from build123d import *

# Parameters (mm, degrees)
SKETCH2_W           = 26
SKETCH2_H           = 11
SKETCH2_W_2         = 20.4
SKETCH2_H_2         = 6.5
BOSS_EXTRUDE1_DEPTH = 10
SKETCH3_W           = 26
SKETCH3_H           = 11
SKETCH3_W_2         = 2.5
SKETCH3_H_2         = 6.5
BOSS_EXTRUDE2_DEPTH = 6
SKETCH4_W           = 11
SKETCH4_H           = 40
SKETCH4_R           = 2.85
BOSS_EXTRUDE3_DEPTH = 6
FILLET1_R           = 2


with BuildPart() as part:
    # Sketch2 → Boss-Extrude1 (new body)
    with BuildSketch(Plane(origin=(0, 0, 0), x_dir=(1, 0, 0), z_dir=(0, 1, 0))):
        Rectangle(SKETCH2_W, SKETCH2_H)
        Rectangle(SKETCH2_W_2, SKETCH2_H_2, mode=Mode.SUBTRACT)
    extrude(amount=BOSS_EXTRUDE1_DEPTH)

    # Sketch3 → Boss-Extrude2 (add)
    with BuildSketch(Plane.XZ):
        Rectangle(SKETCH3_W, SKETCH3_H)
        with Locations((-7.45, 0)):
            Rectangle(SKETCH3_W_2, SKETCH3_H_2, mode=Mode.SUBTRACT)
        with Locations((-0.25, 0)):
            Rectangle(SKETCH3_W_2, SKETCH3_H_2, mode=Mode.SUBTRACT)
        with Locations((7.45, 0)):
            Rectangle(SKETCH3_W_2, SKETCH3_H_2, mode=Mode.SUBTRACT)
    extrude(amount=BOSS_EXTRUDE2_DEPTH)

    # Sketch4 → Boss-Extrude3 (add)
    with BuildSketch(Plane(origin=(13, 0, 0), x_dir=(0, 0, -1), z_dir=(1, 0, 0))):
        with Locations((0, 2)):
            Rectangle(SKETCH4_W, SKETCH4_H)
        with Locations((0, 16)):
            Circle(SKETCH4_R, mode=Mode.SUBTRACT)
        with Locations((0, -11.995757917)):
            Circle(SKETCH4_R, mode=Mode.SUBTRACT)
    extrude(amount=BOSS_EXTRUDE3_DEPTH)

    # Fillet1
    fillet1_edges = [part.edges().sort_by_distance(p)[0] for p in [
        (13, -6, 0),
        (13, 10, 0),
    ]]
    fillet(fillet1_edges, radius=FILLET1_R)


solid = part.part
Can you work these out from the model? Positions are in its coordinate system, mm. A direction names the side the tool comes from. Round coordinates to 2 decimals unless told otherwise and drop trailing zeros. Loops run counter-clockwise (first coordinate to the right, second up) from the corner with the lowest first, then second, coordinate; pieces in that order, holes last. Notation, with made-up numbers: (-37, 32.5) - (-18, 32.5) arc R19 cw to (-18, 67.5) - close; hole circle Ø2 at (10.25, 71). An arc over 180 degrees is marked (long way). Write item = value, one per line. Start each with the question number.
(1) If we section it at B-B (z = 0): Give the number of separate pieces and of enclosed holes in the cut face, and give its area (3 significant figures).
(2) If we section it at A-A (y = 16): Please give me the cut outline in (x, z).
(3) For P1, Ø3, axis at y = -14, z = -2.5, coming from the -X side; P2, Ø2, axis at x = 10, z = -3, coming from the +Y side; P3, Ø2.5, axis at x = -4.5, z = 0.5, coming from the +Y side, each with a flat end and sliding along its axis, tell me the tip position at first contact or that it passes through.
(4) If I drill on probe 1 along Y at (x, z) = (16.65, 0); probe 2 along X at (y, z) = (-3, 2.5); probe 3 along X at (y, z) = (2, -3), over which ranges is the centre line in solid material (lowest first)? Write a range as [from, to].
(5) If we mould it in two halves opening along Z, with no side actions, what happens to faces 4 (the face through (15.958, 18.403, -1.532)), 5 (the face through (6, 2, 5.5)), 6 (the face through (12.43, 10.6, -0.08))? For each: released by +Z, released by -Z, zero draft, split by the parting line, or undercut.
(6) For faces 1 (the face through (9, 0, 0)), 2 (the face through (13, -15, 0)), 3 (the face through (8.7, -3, 0)), which set-ups out of +Z, -Z, +X, -X, +Y, -Y let a thin tool reach every point of the face, with its end or its side?
(7) If we section it at D-D (x = -3): Please give me the cut outline in (y, z).
(8) If we section it at C-C (x = -8): Please give me the cut outline in (y, z).
Ans:
q1.separate_pieces = 6
q1.enclosed_holes = 0
q1.area = 340 mm²
q2.outline = (13, -5.5) - (19, -5.5) - (19, -2.85) - (13, -2.85) - close; (13, 2.85) - (19, 2.85) - (19, 5.5) - (13, 5.5) - close
q3.P1 = 13
q3.P2 = 10
q3.P3 = 0
q4.probe_1 = [-18, -14.85], [-9.15, 13.15], [18.85, 22]
q4.probe_2 = [-13, -8.7], [-6.2, -1.5], [1, 6.2], [8.7, 19]
q4.probe_3 = [-13, -10.2], [10.2, 19]
q5.face_4 = undercut
q5.face_5 = released by +Z
q5.face_6 = zero draft
q6.face_1 = +Y
q6.face_2 = +Z, -Z, -X, -Y
q6.face_3 = +Y, -Y
q7.outline = (-6, -5.5) - (10, -5.5) - (10, -3.25) - (0, -3.25) - (0, 3.25) - (10, 3.25) - (10, 5.5) - (-6, 5.5) - close
q8.outline = (-6, -5.5) - (10, -5.5) - (10, -3.25) - (-6, -3.25) - close; (-6, 3.25) - (10, 3.25) - (10, 5.5) - (-6, 5.5) - close
